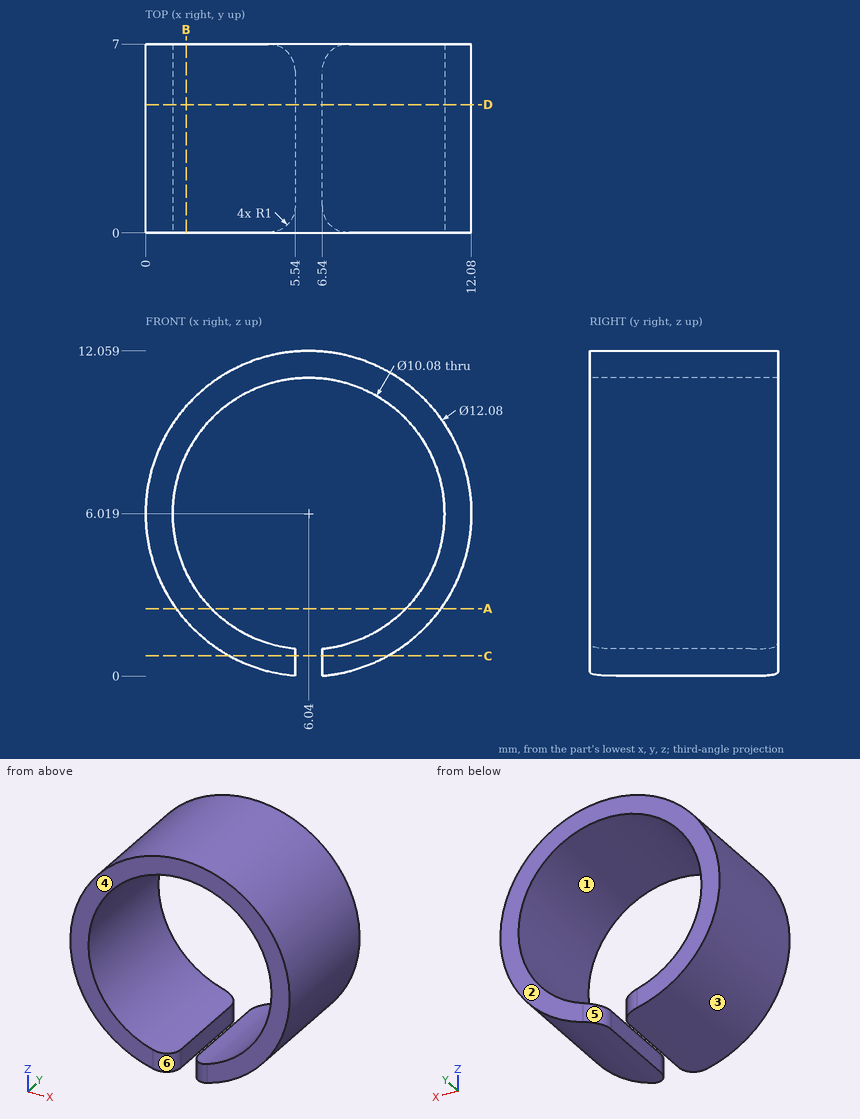
The figure shows three views and two pictorial views of one solid part (mm, origin at its lowest corner). Answer the questions. A direction names the side the tool comes from. Round coordinates to 2 decimals unless told otherwise and drop trailing zeros. Write each loop counter-clockwise with the first axis right and the second up, starting at its lowest first coordinate (ties: lowest second). Pieces come first, ordered by that corner, then holes. Notation, with made-up numbers: (-15, 38) - (24, 38) arc R23 ccw to (24, 72) - close; hole circle Ø7 at (63.5, 56). An arc over 180 degrees is marked (long way). One line per question, with ' | ' between items. Start each with the question number.
1. Find the intervals of material crossed by probe 1 along X at (y, z) = (3, 1.75); probe 2 along Z at (x, y) = (8.5, 2) (1 decimal); probe 3 along X at (y, z) = (4.5, 5), in increasing order. Write a range as [from, to].
2. Each of these flat-tipped pins is pushed along its axis until it touches: pin 1 (0.8 mm diameter, centred on y = 4.5, z = 0.5, fed in from +X) (1 decimal); pin 2 (3 mm diameter, centred on y = 4, z = 7.5, fed in from +X); pin 3 (4 mm diameter, centred on y = 1.5, z = 1.5, fed in from -X); pin 4 (0.8 mm diameter, centred on y = 3.5, z = 0.5, fed in from -X) (1 decimal). Where does it stop, or does it pass through?
3. For a pull along X with two mould halves and no side action, classify the marked faces 1, 2 and 3 as +X half, -X half, draft (parallel to the pull), parting line (faces both ways), or undercut.
4. Section D-D (y = 4.75) is taken. Determine the outline of the cut face in (x, z), and give its area (3 significant figures).
5. Section A-A (z = 2.5) is taken. Determine the outline of the cut face in (x, y), and give its area (3 significant figures).
6. For the marked faces 4, 5 and 6, determine the directions among +Z, -Z, +X, -X, +Y, -Y from which every point of the face is accessible in a straight line to the end or side of a thin tool.
7. Section C-C (z = 0.75) is taken. Determine the outline of the cut face in (x, y), and give its area (3 significant figures).
8. Section B-B (x = 1.5) is taken. Determine the outline of the cut face in (y, z).
Filled in:
1) probe 1: [1.77, 3.36], [8.72, 10.31] | probe 2: [0.5, 1.6], [10.4, 11.5] | probe 3: [0.09, 1.1], [10.98, 11.99]
2) pin 1: x = 9.2 | pin 2: x = 12.08 | pin 3: x = 0.55 | pin 4: x = 2.8
3) face 1: undercut | face 2: draft | face 3: parting line
4) outline: (5.54, 0) - (5.54, 1) arc R5.04 cw (long way) to (6.54, 1) - (6.54, 0) arc R6.04 ccw (long way) to start | area: 33.8 mm²
5) outline: (1.13, 0) - (2.43, 0) - (2.43, 7) - (1.13, 7) - close; (9.65, 0) - (10.95, 0) - (10.95, 7) - (9.65, 7) - close | area: 18.2 mm²
6) face 4: +Z, -Z, +X, -X, -Y | face 5: -Z, +Y | face 6: -Z, -Y
7) outline: (3.09, 0) - (4.54, 0) arc R1 ccw to (5.54, 1) - (5.54, 6) arc R1 ccw to (4.54, 7) - (3.09, 7) - close; (6.54, 1) arc R1 ccw to (7.54, 0) - (8.99, 0) - (8.99, 7) - (7.54, 7) arc R1 ccw to (6.54, 6) - close | area: 33.5 mm²
8) outline: (0, 2.04) - (7, 2.04) - (7, 3.83) - (0, 3.83) - close; (0, 8.21) - (7, 8.21) - (7, 10) - (0, 10) - close
